For this review, take the finished solid that the model builds, in its own axes (mm). A direction names the side the tool comes from. Give positions to 0.01 mm unless a question says otherwise; leave off trailing zeros. Order: outer loops, then holes, each group sorted by start corner. A loop starts at its lowest first (then second) coordinate and runs counter-clockwise, first axis right, second up.
from build123d import *

# Parameters (mm, degrees)
F1_DEPTH = 24
F2_DEPTH = 22.75
F3_R     = 5
F4_DEPTH = 42.5
F5_R     = 1.65
F6_DEPTH = 25
F7_START = 2
F5_R_2   = 3.75
F7_DEPTH = 23
F9_DEPTH = 1


with BuildPart() as f1:
    # F0 (on Front) → F1 (new body, symmetric)
    with BuildSketch(Plane.XZ):
        with BuildLine():
            ThreePointArc((-24.1761827572, 27.2544863717), (-26.8028128996, 25.4428226271), (-27.6068595339, 22.3549721713))
            Line((-27.6068595339, 22.3549721713), (-25.9186847038, 24.76593569))
            Line((-25.9186847038, 24.76593569), (-24.1761827572, 27.2544863717))
        make_face()
        with BuildLine():
            Line((-33, 4), (-15.9628038305, 4))
            Line((-15.9628038305, 4), (-31.2942431747, 14.7351894004))
            Line((-31.2942431747, 14.7351894004), (-32.4000984345, 15.5095175895))
            add(Edge.make_bspline(
                [(-32.4000984345, 15.5095175895), (-33.6793400347, 13.5531779379), (-33, 7.9824011773), (-33, 4)],
                knots=[0, 0, 0, 0, 11.5251410851, 11.5251410851, 11.5251410851, 11.5251410851], degree=3))
        make_face()
        Polygon((-33, 0), (-10.2502118035, 0), (-15.9628038305, 4), (-33, 4), align=None)
        Polygon((-9.8717945621, 0), (0, 0), (0, 4), (-7.0709644092, 4), align=None)
        Polygon((-1.1058552598, 12.5190587418), (-1.7330256341, 11.6233666218), (-2.2487850863, 9.0910355887), (-0.2621286542, 11.9282750123), align=None)
        Polygon((-7.0709644092, 4), (0, 4), (0, 7.8723652764), (0, 11.7447305527), (-0.2621286542, 11.9282750123), (-2.2487850863, 9.0910355887), (-2.4090210327, 8.3042919667), (-5.1744842522, 6.7084543561), align=None)
        Polygon((-15.9628038305, 4), (-7.0709644092, 4), (-5.1744842522, 6.7084543561), (-1.7330256341, 11.6233666218), (-1.1058552598, 12.5190587418), (-22.4038084113, 27.4320460869), (-23.0309787856, 26.5363539669), (-26.4724374037, 21.6214417012), (-31.2942431747, 14.7351894004), align=None)
        Polygon((-1.7330256341, 11.6233666218), (-5.1744842522, 6.7084543561), (-2.4090210327, 8.3042919667), (-2.2487850863, 9.0910355887), align=None)
        Polygon((-10.2502118035, 0), (-9.8717945621, 0), (-7.0709644092, 4), (-15.9628038305, 4), align=None)
        Polygon((-25.9186847038, 24.76593569), (-26.4724374037, 21.6214417012), (-23.0309787856, 26.5363539669), (-25.2341914491, 25.1855903927), align=None)
        Polygon((-32.4000984345, 15.5095175895), (-31.2942431747, 14.7351894004), (-26.4724374037, 21.6214417012), (-25.9186847038, 24.76593569), (-27.6068595339, 22.3549721713), align=None)
        Polygon((-24.1761827572, 27.2544863717), (-25.9186847038, 24.76593569), (-25.2341914491, 25.1855903927), (-23.2475350169, 28.0228298164), (-23.5096636711, 28.206374276), align=None)
        Polygon((-25.2341914491, 25.1855903927), (-23.0309787856, 26.5363539669), (-22.4038084113, 27.4320460869), (-23.2475350169, 28.0228298164), align=None)
    extrude(amount=F1_DEPTH, both=True)

    # F0 (on Front) → F2 (cut, symmetric)
    with BuildSketch(Plane.XZ):
        Polygon((-15.9628038305, 4), (-7.0709644092, 4), (-5.1744842522, 6.7084543561), (-1.7330256341, 11.6233666218), (-1.1058552598, 12.5190587418), (-22.4038084113, 27.4320460869), (-23.0309787856, 26.5363539669), (-26.4724374037, 21.6214417012), (-31.2942431747, 14.7351894004), align=None)
        Polygon((-25.9186847038, 24.76593569), (-26.4724374037, 21.6214417012), (-23.0309787856, 26.5363539669), (-25.2341914491, 25.1855903927), align=None)
        Polygon((-1.7330256341, 11.6233666218), (-5.1744842522, 6.7084543561), (-2.4090210327, 8.3042919667), (-2.2487850863, 9.0910355887), align=None)
        Polygon((-10.2502118035, 0), (-9.8717945621, 0), (-7.0709644092, 4), (-15.9628038305, 4), align=None)
        Polygon((-25.2341914491, 25.1855903927), (-23.0309787856, 26.5363539669), (-22.4038084113, 27.4320460869), (-23.2475350169, 28.0228298164), align=None)
        Polygon((-1.1058552598, 12.5190587418), (-1.7330256341, 11.6233666218), (-2.2487850863, 9.0910355887), (-0.2621286542, 11.9282750123), align=None)
    extrude(amount=F2_DEPTH, both=True, mode=Mode.SUBTRACT)

    # F3 (on face) → F4 (cut)
    with BuildSketch(Plane(origin=(0, 24, 0), x_dir=(-1, 0, 0), z_dir=(0, 1, 0))):
        with Locations((24, 9)):
            Circle(F3_R)
    extrude(amount=-F4_DEPTH, mode=Mode.SUBTRACT)

    # F5 (on Top) → F6 (cut)
    with BuildSketch(Plane.XY):
        with Locations((-20.7403171808, 0)):
            Circle(F5_R)
    extrude(amount=F6_DEPTH, mode=Mode.SUBTRACT)

    # F5 (on Top) → F7 (cut)
    with BuildSketch(Plane.XY.offset(F7_START)):
        with Locations((-20.7403171808, 0)):
            Circle(F5_R_2)
        with Locations((-20.7403171808, 0)):
            Circle(F5_R, mode=Mode.SUBTRACT)
    extrude(amount=F7_DEPTH, mode=Mode.SUBTRACT)

    # F8 (on face) → F9 (join)
    with BuildSketch(Plane.YZ):
        Polygon((-7.1003163303, 9.557886192), (-11.4740050518, 0), (-8.8921013951, 0), (-4.4878274378, 10.0829327401), (-4.4878274378, 11.6300359184), (-12.8426943545, 11.6300359184), (-12.8426943545, 9.557886192), align=None)
        with BuildLine():
            Line((-3.3179421679, 1.7127732056), (-3.3179421679, 0))
            Line((-3.3179421679, 0), (4.822828098, 0))
            Line((4.822828098, 0), (4.822828098, 2.0721497264))
            Line((4.822828098, 2.0721497264), (-0.2517722775, 2.0721497264))
            Line((-0.2517722775, 2.0721497264), (-0.2517722775, 2.1817468214))
            Line((-0.2517722775, 2.1817468214), (1.2469042774, 3.5912164385))
            add(Edge.make_bspline(
                [(3.3368953913, 5.7028720946), (2.7430320626, 4.9624545109), (1.2469042774, 3.5912164385)],
                knots=[0, 0, 0, 1, 1, 1], degree=2))
            add(Edge.make_bspline(
                [(4.2136721514, 7.1480244868), (3.9307587201, 6.4432896782), (3.3368953913, 5.7028720946)],
                knots=[0, 0, 0, 1, 1, 1], degree=2))
            add(Edge.make_bspline(
                [(4.4965855826, 8.6581705051), (4.4965855826, 7.8527592953), (4.2136721514, 7.1480244868)],
                knots=[0, 0, 0, 1, 1, 1], degree=2))
            add(Edge.make_bspline(
                [(4.0339838909, 10.2983037757), (4.4965855826, 9.5808251188), (4.4965855826, 8.6581705051)],
                knots=[0, 0, 0, 1, 1, 1], degree=2))
            add(Edge.make_bspline(
                [(2.7353857537, 11.4133904981), (3.5713821992, 11.0157824325), (4.0339838909, 10.2983037757)],
                knots=[0, 0, 0, 1, 1, 1], degree=2))
            add(Edge.make_bspline(
                [(1.6567308132, 11.7447305527), (2.2406834278, 11.6486757506), (2.7353857537, 11.4133904981)],
                knots=[0.4082482905, 0.4082482905, 0.4082482905, 1, 1, 1], degree=2))
            Line((1.6567308132, 11.7447305527), (-0.1827126259, 11.7447305527))
            add(Edge.make_bspline(
                [(-0.6888862727, 11.647877306), (-0.4462729111, 11.7070287542), (-0.1827126259, 11.7447305527)],
                knots=[0, 0, 0, 0.3626225608, 0.3626225608, 0.3626225608], degree=2))
            add(Edge.make_bspline(
                [(-1.9237651687, 11.1827268446), (-1.3579383062, 11.4847560483), (-0.6888862727, 11.647877306)],
                knots=[0, 0, 0, 1, 1, 1], degree=2))
            add(Edge.make_bspline(
                [(-3.3485274038, 10.1466519814), (-2.4895920313, 10.880697641), (-1.9237651687, 11.1827268446)],
                knots=[0, 0, 0, 1, 1, 1], degree=2))
            Line((-3.3485274038, 10.1466519814), (-2.0104233369, 8.5613172584))
            add(Edge.make_bspline(
                [(-0.6799655789, 9.4457403273), (-1.3171579917, 9.1347904299), (-2.0104233369, 8.5613172584)],
                knots=[0, 0, 0, 1, 1, 1], degree=2))
            add(Edge.make_bspline(
                [(0.6326507914, 9.7566902248), (-0.0427731661, 9.7566902248), (-0.6799655789, 9.4457403273)],
                knots=[0, 0, 0, 1, 1, 1], degree=2))
            add(Edge.make_bspline(
                [(1.6649025002, 9.4138807067), (1.2774895132, 9.7566902248), (0.6326507914, 9.7566902248)],
                knots=[0, 0, 0, 1, 1, 1], degree=2))
            add(Edge.make_bspline(
                [(2.0523154871, 8.3701595345), (2.0523154871, 9.0710711886), (1.6649025002, 9.4138807067)],
                knots=[0, 0, 0, 1, 1, 1], degree=2))
            add(Edge.make_bspline(
                [(1.8764503812, 7.4627975387), (2.0523154871, 7.9011859187), (2.0523154871, 8.3701595345)],
                knots=[0, 0, 0, 1, 1, 1], degree=2))
            add(Edge.make_bspline(
                [(1.3029772097, 6.510832074), (1.7005852753, 7.0244091587), (1.8764503812, 7.4627975387)],
                knots=[0, 0, 0, 1, 1, 1], degree=2))
            add(Edge.make_bspline(
                [(-0.394503378, 4.6667972313), (0.9053691441, 5.9972549893), (1.3029772097, 6.510832074)],
                knots=[0, 0, 0, 1, 1, 1], degree=2))
            Line((-0.394503378, 4.6667972313), (-3.3179421679, 1.7127732056))
        make_face()
        with BuildLine():
            Line((5.3402283372, 8.9054011613), (8.7326407429, 0))
            Line((8.7326407429, 0), (11.2253374618, 0))
            Line((11.2253374618, 0), (14.6202986372, 8.9054011613))
            Line((14.6202986372, 8.9054011613), (12.0791752949, 8.9054011613))
            Line((12.0791752949, 8.9054011613), (10.3664020893, 3.8308007857))
            add(Edge.make_bspline(
                [(10.0070255685, 2.0084304851), (10.0478058829, 2.7730613805), (10.3664020893, 3.8308007857)],
                knots=[0, 0, 0, 1, 1, 1], degree=2))
            Line((10.0070255685, 2.0084304851), (9.9611477148, 2.0084304851))
            add(Edge.make_bspline(
                [(9.601771194, 3.8308007857), (9.8872333949, 2.8673658576), (9.9611477148, 2.0084304851)],
                knots=[0, 0, 0, 1, 1, 1], degree=2))
            Line((9.601771194, 3.8308007857), (7.8813516794, 8.9054011613))
            Line((7.8813516794, 8.9054011613), (5.3402283372, 8.9054011613))
        make_face()
    extrude(amount=F9_DEPTH)


solid = f1.part
1) We need section B-B on z = 18.5. Give the boundary of the cut face in (x, y).
Answer sheet:
outline: (-30.31, -24) - (-9.65, -24) - (-9.65, -22.75) - (-28.66, -22.75) - (-28.66, 22.75) - (-9.65, 22.75) - (-9.65, 24) - (-30.31, 24) - close
2) Tool access review of faces 4 (the face through (0.5, 2.3, 2.072)), 5 (the face through (0.493, 11.235, 6.404)), 6 (the face through (-33, 0, 2)): name each direction out of +Z, -Z, +X, -X, +Y, -Y from which nothing blocks a thin tool from reaching the whole face with its end or side.
Answer sheet:
face 4: +X
face 5: +Z, +X
face 6: -Z, -X, +Y, -Y
3) Draft analysis for pull direction Y (two halves, no side actions). For faces 1 (the face through (-19, -1, 2)), 2 (the face through (0.49, 12.9, 4.39)), 3 (the face through (1, 1, 5)), state which applies: +Y half, -Y half, draft (parallel to the pull), parting line (faces both ways), or undercut.
Answer sheet:
face 1: undercut
face 2: +Y half
face 3: draft
4) We need section A-A on x = -20.5. Give the boundary of the cut face in (y, z).
Answer sheet:
outline: (-24, 0) - (-1.63, 0) - (-1.63, 2) - (-3.74, 2) - (-3.74, 5.43) - (-18.5, 5.43) - (-18.5, 7.18) - (-22.75, 7.18) - (-22.75, 26.1) - (-24, 26.1) - close; (1.63, 0) - (24, 0) - (24, 5.43) - (3.74, 5.43) - (3.74, 2) - (1.63, 2) - close; (22.75, 12.57) - (24, 12.57) - (24, 26.1) - (22.75, 26.1) - close
5) To check wall thickness, follow line 1 (Y direction, x = -7.5, z = 6.5); line 2 (Y direction, x = -25, z = 4.75); line 3 (X direction, y = 13, z = 9). State the ranges of each line that lie inside material, in increasing order.
Answer sheet:
line 1: y = -24 to -22.75, 22.75 to 24
line 2: y = -24 to -18.5
line 3: x = -33.15 to -29, -2.27 to 0
6) Clearance check with flat-ended pins moving along their axes: pin 1 (5 mm diameter, centred on y = 16, z = 3, fed in from +X); pin 2 (4 mm diameter, centred on y = 13, z = 24.5, fed in from -X); pin 3 (4.5 mm diameter, centred on y = -10, z = 1.5, fed in from -X). State where each tip first meets the part, or that it passes through.
Answer sheet:
pin 1: stops at x = 0
pin 2: stops at x = -27.63
pin 3: stops at x = -33
7) We need section C-C on x = -13. Give the boundary of the cut face in (y, z).
Answer sheet:
outline: (-24, 0) - (24, 0) - (24, 20.85) - (22.75, 20.85) - (22.75, 1.93) - (-22.75, 1.93) - (-22.75, 20.85) - (-24, 20.85) - close
